Autodesk Inventor part; units mm, degrees
ref_plane "YZ Plane" through (0, 0, 0) normal (1, 0, 0) x (0, 1, 0)
ref_plane "XZ Plane" through (0, 0, 0) normal (0, 1, 0) x (-1, 0, 0)
ref_plane "XY Plane" through (0, 0, 0) normal (0, 0, 1) x (1, 0, 0)
sketch "Sketch1" plane through (0, 0, 0) normal (0, 1, 0) x (-1, 0, 0)
  line L0 (0, 0) -> (104.9602, 0)
  line L1 (104.9602, 0) -> (104.9602, -450.85)
  line L2 (104.9602, -450.85) -> (38.1, -450.85)
  line L3 (0, -412.75) -> (0, 0)
  arc A0 (0, -412.75) -> (38.1, -450.85) centre (38.1, -412.75) ccw
  line L4 (38.1, -412.75) -> (38.1, -450.85) construction
  line L5 (38.1, -412.75) -> (76.2, -412.75) construction
  dimension "d1" = 450.85
  dimension "d5" = 38.1
  dimension "d6" = 90
  dimension "d7" = 104.9602
  dimension "d8" = 38.1
extrude "Extrusion1" add sketch "Sketch1" along normal blind 5
sketch "Sketch2" plane through (0, 5, 0) normal (0, 1, 0) x (1, 0, 0)
  circle A0 centre (-31.75, 57.3786) radius 6.95
  line L0 (-104.9602, 0) -> (0, 0)
  line L1 (0, 0) -> (0, 412.75)
  circle A1 centre (-31.75, 393.4714) radius 6.95
  circle A2 centre (-6.35, 6.35) radius 2.15
  dimension "BearingHole" = 13.9
  dimension "d12" = 57.3786
  dimension "d13" = 31.75
  dimension "d14" = 13.9
  dimension "d15" = 31.75
  dimension "d16" = 336.0928
  dimension "M4Clearance" = 4.3
  dimension "d71" = 6.35
  dimension "d72" = 6.35
extrude "Extrusion2" cut sketch "Sketch2" against normal through all
sketch "Sketch3" plane through (0, 5, 0) normal (0, 1, 0) x (1, 0, 0)
  circle A0 centre (-97.3271, 444.4951) radius 1.7 construction
  circle A1 centre (-97.3271, 6.3451) radius 1.7 construction
  circle A2 centre (-63.6771, 179.4396) radius 3.15 construction
  circle A3 centre (-95.6771, 179.4396) radius 3.5 construction
  circle A4 centre (-79.6771, 147.4247) radius 7 construction
  circle A5 centre (-31.6771, 291.4544) radius 7 construction
  circle A6 centre (-15.6771, 259.4396) radius 3.5 construction
  circle A7 centre (-47.6771, 259.4396) radius 3.5 construction
  circle A8 centre (-31.75, 393.4714) radius 6.95 construction
  circle A9 centre (-15.6771, 163.4396) radius 2.25 construction
  arc A10 (-33.6771, 302.7533) -> (-29.6771, 302.7533) centre (-31.6771, 302.7533) ccw construction
  arc A11 (-29.6771, 304.1259) -> (-33.6771, 304.1259) centre (-31.6771, 304.1259) ccw construction
  line L0 (-29.6771, 302.7533) -> (-29.6771, 304.1259) construction
  line L1 (-33.6771, 304.1259) -> (-33.6771, 302.7533) construction
  line L2 (-77.6771, 158.7533) -> (-77.6771, 160.1259) construction
  arc A12 (-77.6771, 160.1259) -> (-81.6771, 160.1259) centre (-79.6771, 160.1259) ccw construction
  line L3 (-81.6771, 160.1259) -> (-81.6771, 158.7533) construction
  arc A13 (-81.6771, 158.7533) -> (-77.6771, 158.7533) centre (-79.6771, 158.7533) ccw construction
  circle A14 centre (-97.3271, 6.3451) radius 1.65
  circle A15 centre (-97.3271, 444.4951) radius 1.65
  circle A16 centre (-79.6771, 147.4247) radius 6.95
  circle A17 centre (-31.6771, 291.4544) radius 6.95
  circle A18 centre (-15.6771, 163.4396) radius 2.413
  arc A19 (-77.6771, 136.1259) -> (-81.6771, 136.1259) centre (-79.6771, 136.1259) ccw construction
  line L4 (-77.6771, 134.7533) -> (-77.6771, 136.1259) construction
  line L5 (-81.6771, 136.1259) -> (-81.6771, 134.7533) construction
  arc A20 (-81.6771, 134.7533) -> (-77.6771, 134.7533) centre (-79.6771, 134.7533) ccw construction
  circle A21 centre (-90.4602, 355.95) radius 1.7 construction
  circle A22 centre (-90.4602, 355.95) radius 1.65
  circle A23 centre (-90.4602, 101.631) radius 1.7 construction
  circle A24 centre (-90.4602, 101.631) radius 1.65
  point P0 (0, 0)
  dimension "d75" = 3.3
  dimension "d76" = 3.3
  dimension "BearingClearance" = 13.9
  dimension "d78" = 13.9
  dimension "d83" = 4.826
  dimension "d90" = 3.3
  dimension "d91" = 3.3
extrude "Extrusion3" cut sketch "Sketch3" against normal through all
sketch "Sketch4" plane through (0, 0, 0) normal (0, -1, 0) x (1, 0, 0)
  circle A0 centre (-73.66, -342.8852) radius 1.7 construction
  circle A1 centre (-95.6771, -203.4396) radius 1.9304 construction
  circle A2 centre (-47.6771, -227.4396) radius 1.9304 construction
  circle A3 centre (-15.6771, -227.4396) radius 1.9304 construction
  circle A4 centre (-54.3045, -291.4544) radius 2 construction
  circle A5 centre (-95.6771, -283.4396) radius 1.9304 construction
  circle A6 centre (-63.6771, -203.4396) radius 1.9304 construction
  circle A7 centre (-63.6771, -203.4396) radius 1.9304 construction
  circle A8 centre (-15.6771, -147.4396) radius 1.9304 construction
  circle A9 centre (-73.66, -342.8852) radius 1.65
  circle A10 centre (-95.6771, -283.4396) radius 1.65
  circle A11 centre (-47.6771, -227.4396) radius 1.65
  circle A12 centre (-15.6771, -227.4396) radius 1.65
  circle A13 centre (-95.6771, -203.4396) radius 1.65
  circle A14 centre (-63.6771, -203.4396) radius 1.65
  circle A15 centre (-15.6771, -147.4396) radius 1.65
  point P0 (0, 0)
  dimension "d92" = 3.3
  dimension "d93" = 3.3
  dimension "d94" = 3.3
  dimension "d95" = 3.3
  dimension "d96" = 3.3
  dimension "d97" = 3.3
  dimension "d98" = 3.3
extrude "Extrusion4" cut sketch "Sketch4" against normal through all
sketch "Sketch5" plane through (0, 0, 0) normal (0, -1, 0) x (1, 0, 0)
  circle A0 centre (-90.9801, -147.4247) radius 2
  circle A1 centre (-79.6771, -147.4247) radius 6.95
  circle A2 centre (-20.3741, -291.4544) radius 2
  circle A3 centre (-31.6771, -291.4544) radius 6.95
  point P0 (0, 0)
  dimension "d101" = 4
  dimension "d102" = 11.303
  dimension "d103" = 4
  dimension "d104" = 11.303
extrude "Extrusion5" cut sketch "Sketch5" against normal through all contours A0 | A2
equation "\"d14\" = BearingHole"
equation "\"d15\" = d13"
equation "\"d75\" = M3Clearance"
equation "\"d76\" = M3Clearance"
equation "\"BearingClearance\" = BearingHole"
equation "\"d78\" = BearingHole"
equation "\"d90\" = M3Clearance"
equation "\"d91\" = M3Clearance"
equation "\"d92\" = M3Clearance"
equation "\"d93\" = M3Clearance"
equation "\"d94\" = M3Clearance"
equation "\"d95\" = M3Clearance"
equation "\"d96\" = M3Clearance"
equation "\"d97\" = M3Clearance"
equation "\"d98\" = M3Clearance"
equation "\"d103\" = d101"
equation "\"d104\" = d102"
properties part number "sidewall outside"
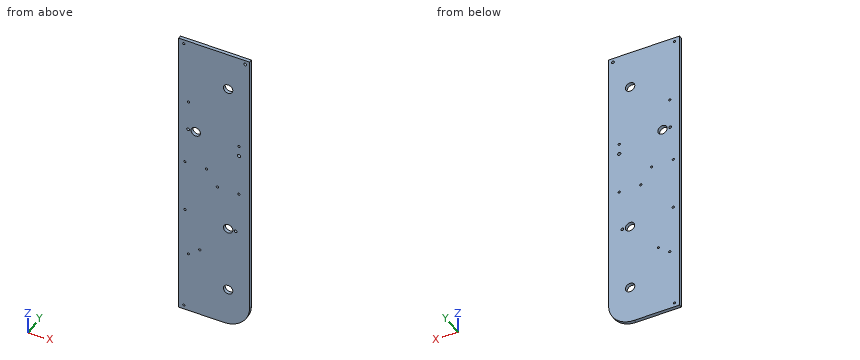
Check sheet for the modelled part. Datum: model origin and axes. Units: mm. Round coordinates to 2 decimals unless told otherwise and drop trailing zeros. Order: outer loops, then holes, each group sorted by start corner. A loop starts at its lowest first (then second) coordinate and runs counter-clockwise, first axis right, second up. Notation, with made-up numbers: (36, 0.25) -> (47, 0.25) arc R25 cw to (47, 29.25) -> close; hole circle Ø4 at (64, 70.5). An arc over 180 degrees is marked (long way). One line per item, written item: value. Start each with the question number.
Q1. Gauge pin test, flat end, axial feed: pin 1 Ø6 at (x, z) = (-63.5, -220.5) entering from -Y. Record the tip position at first contact, or that the pin passes through.
Q2. Cross-section at B-B (y = 0.75). Give the number of separate pieces and of enclosed holes in the cut face, and give its area (3 significant figures).
Q3. Thickness scan on line 1 (Z direction, x = -89.5, y = 2.9); line 2 (Z direction, x = -31.75, y = 1.05); line 3 (Z direction, x = -75.5, y = 4.45). Record the ranges inside material, lowest first.
Q4. Cross-section at A-A (x = -31.75). Record the boundary of the cut face in (y, z).
Completed:
1. pin 1: stops at y = 0
2. separate pieces: 1
2. enclosed holes: 19
2. area: 46,300 mm²
3. line 1: z = -450.85 to -357.29, -354.61 to -148.77, -146.08 to -102.97, -100.29 to 0
3. line 2: z = -450.32 to -400.42, -386.52 to -298.4, -284.5 to -64.33, -50.43 to 0
3. line 3: z = -450.85 to -152.98, -141.87 to 0
4. outline: (0, -450.32) -> (5, -450.32) -> (5, -400.42) -> (0, -400.42) -> close; (0, -386.52) -> (5, -386.52) -> (5, -298.4) -> (0, -298.4) -> close; (0, -284.5) -> (5, -284.5) -> (5, -64.33) -> (0, -64.33) -> close; (0, -50.43) -> (5, -50.43) -> (5, 0) -> (0, 0) -> close
